Geometry: final body of the model. Coordinates: model frame, mm. Face numbers are marked on the shaded views. A direction names the side the tool comes from. Give positions to 0.01 mm unless a question says otherwise; leave off trailing zeros. Order: outer loops, then holes, each group sorted by start corner. A loop starts at its lowest first (then second) coordinate and runs counter-clockwise, first axis right, second up. Notation, with made-up numbers: (36, -4.5) -> (52, -4.5) arc R17 ccw to (52, 0.5) -> close; hole circle Ø9 at (37.25, -5). An arc over 180 degrees is marked (long way). One line per question, with ' | ' between items. Start each with the question number.
(1) Section C-C (x = 0). Return loops of the section in (y, z).
(2) First-contact query: pin 1 Ø1.5 at (x, z) = (25, 6.5) entering from -Y; pin 2 Ø3 at (y, z) = (48.5, 6.5) entering from +X; pin 3 Ø3 at (y, z) = (-2.5, 2.5) entering from -X. Flat tips, straight axial feed; report the tip coordinate or a pass-through.
(3) Section A-A (y = 33). Return loops of the section in (x, z).
(4) Ray query, L1, parallel to Y at x = 0, z = 4.5; L2, parallel to Y at x = 35, z = 5.5; L3, parallel to Y at x = 34.5, z = 7. Return the intervals inside material, ascending.
(5) Section D-D (x = 35). Return loops of the section in (y, z), then the cut area to 3 significant figures.
(6) Section B-B (z = 6.75). State how many separate pieces and enclosed holes the cut face has, then the cut area to 3 significant figures.
(7) Set-up query: the marked faces 1 and 2. Return all of +Z, -Z, +X, -X, +Y, -Y with unobstructed straight access to the full face (end or side cutting, diameter ignored); none if empty.
(8) Mould query, pull axis X, two halves, no side actions, for the marked faces 3, 4 and 5. Classes: +X half, -X half, draft (parallel to the pull), parting line (faces both ways), or undercut.
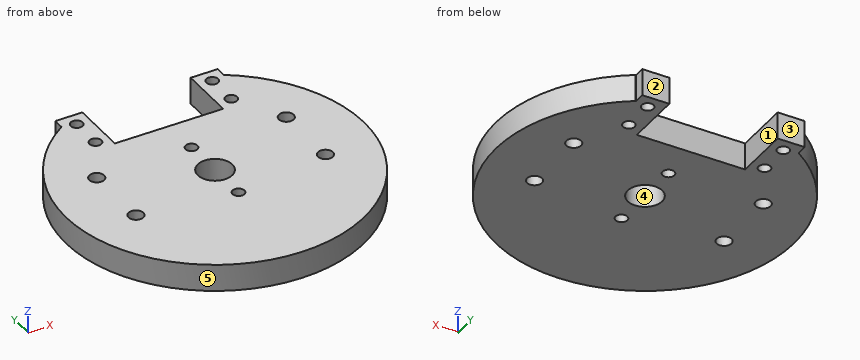
```python
from build123d import *

# Parameters (mm, degrees)
SKETCH1_R           = 55
EXTRUDE_3_8_DEPTH   = 10
CUT_EXTRUDE1_DEPTH  = 10
SKETCH3_W           = 10
SKETCH3_H           = 20.75
BOSS_EXTRUDE2_DEPTH = 10
SKETCH4_R           = 2.2
M4_THROUGH_DEPTH    = 10
SKETCH5_R           = 6.35
CUT_EXTRUDE2_DEPTH  = 10
SKETCH6_R           = 2.2
M4_THROUGH2_DEPTH   = 10
SKETCH7_R           = 2.75
M5_THROUGH_DEPTH    = 10


with BuildPart() as part:
    # Sketch1 → 3/8 (new body)
    with BuildSketch(Plane.XY):
        Circle(SKETCH1_R)
    extrude(amount=EXTRUDE_3_8_DEPTH)

    # Sketch2 → Cut-Extrude1 (cut)
    with BuildSketch(Plane.XY.offset(10)):
        Polygon((-20.05060394, 46), (-20.05060394, 29.25), (19.94939606, 29.25), (19.94939606, 46), (30.149626863, 46), (30.149626863, 76.355115637), (-30.149626863, 76.355115637), (-30.149626863, 46), align=None)
    extrude(amount=-CUT_EXTRUDE1_DEPTH, mode=Mode.SUBTRACT)

    # Sketch3 → Boss-Extrude2 (add)
    with BuildSketch(Plane.XY.offset(10)):
        with Locations((-25.05060394, 39.625)):
            Rectangle(SKETCH3_W, SKETCH3_H)
        with Locations((24.94939606, 39.625)):
            Rectangle(SKETCH3_W, SKETCH3_H)
    extrude(amount=-BOSS_EXTRUDE2_DEPTH)

    # Sketch4 → M4_through (cut)
    with BuildSketch(Plane.XY.offset(10)):
        with Locations((-25.05060394, 45)):
            Circle(SKETCH4_R)
        with Locations((-25.05060394, 33)):
            Circle(SKETCH4_R)
        with Locations((25.05060394, 33)):
            Circle(SKETCH4_R)
        with Locations((25.05060394, 45)):
            Circle(SKETCH4_R)
    extrude(amount=-M4_THROUGH_DEPTH, mode=Mode.SUBTRACT)

    # Sketch5 → Cut-Extrude2 (cut)
    with BuildSketch(Plane.XY.offset(10)):
        Circle(SKETCH5_R)
    extrude(amount=-CUT_EXTRUDE2_DEPTH, mode=Mode.SUBTRACT)

    # Sketch6 → M4_through2 (cut)
    with BuildSketch(Plane.XY.offset(10)):
        with Locations((0, 15)):
            Circle(SKETCH6_R)
        with Locations((0, -15)):
            Circle(SKETCH6_R)
    extrude(amount=-M4_THROUGH2_DEPTH, mode=Mode.SUBTRACT)

    # Sketch7 → M5_through (cut)
    with BuildSketch(Plane.XY.offset(10)):
        with Locations((-35, 15)):
            Circle(SKETCH7_R)
        with Locations((-35, -10)):
            Circle(SKETCH7_R)
        with Locations((35, -10)):
            Circle(SKETCH7_R)
        with Locations((35, 15)):
            Circle(SKETCH7_R)
    extrude(amount=-M5_THROUGH_DEPTH, mode=Mode.SUBTRACT)


solid = part.part
```
Response:
1) outline: (-55, 0) -> (-17.2, 0) -> (-17.2, 10) -> (-55, 10) -> close; (-12.8, 0) -> (-6.35, 0) -> (-6.35, 10) -> (-12.8, 10) -> close; (6.35, 0) -> (12.8, 0) -> (12.8, 10) -> (6.35, 10) -> close; (17.2, 0) -> (29.25, 0) -> (29.25, 10) -> (17.2, 10) -> close
2) pin 1: stops at y = -49.37 | pin 2: stops at x = 29.95 | pin 3: stops at x = -54.99
3) outline: (-44, 0) -> (-27.25, 0) -> (-27.25, 10) -> (-44, 10) -> close; (-22.85, 0) -> (-20.05, 0) -> (-20.05, 10) -> (-22.85, 10) -> close; (19.95, 0) -> (22.85, 0) -> (22.85, 10) -> (19.95, 10) -> close; (27.25, 0) -> (44, 0) -> (44, 10) -> (27.25, 10) -> close
4) L1: y = -55 to -17.2, -12.8 to -6.35, 6.35 to 12.8, 17.2 to 29.25 | L2: y = -42.43 to -12.75, -7.25 to 12.25, 17.75 to 42.43 | L3: y = -42.83 to -12.7, -7.3 to 12.3, 17.7 to 42.83
5) outline: (-42.43, 0) -> (-12.75, 0) -> (-12.75, 10) -> (-42.43, 10) -> close; (-7.25, 0) -> (12.25, 0) -> (12.25, 10) -> (-7.25, 10) -> close; (17.75, 0) -> (42.43, 0) -> (42.43, 10) -> (17.75, 10) -> close | area: 739 mm^2
6) separate pieces: 1 | enclosed holes: 11 | area: 8,230 mm^2
7) face 1: +Z, -Z, +Y | face 2: +Z, -Z, +X, -X, +Y
8) face 3: draft | face 4: undercut | face 5: parting line
